Read the model definition and answer for the solid it produces. Units are mm, in the model's axes. Face numbers are marked on the shaded views. A direction names the side the tool comes from. Coordinates: 2 decimals unless noted, no trailing zeros. Loops run counter-clockwise (first coordinate to the right, second up) from the corner with the lowest first, then second, coordinate; pieces in that order, holes last. Notation, with made-up numbers: (36, 1.5) -> (90, 1.5) arc R12 ccw to (90, 7.5) -> close; hole circle Ø8 at (0.25, 2). An arc over 180 degrees is marked (long way). Answer as a JSON object with one key per item and string values. Group by question number.
1) Section C-C, the plane z = 54 is taken. Give the vertices of the cut face in (x, y).
2) Determine the mould class of the marked faces 4 and 5 for opening direction Y: released by +Y, released by -Y, zero draft, split by the parting line, or undercut.
3) Section A-A, the plane y = -15 is taken. Give the vertices of the cut face in (x, z).
4) Consider probe 1 along Z at (x, y) = (3, -10); probe 2 along Y at (x, z) = (1.5, 76); probe 3 along X at (y, z) = (-70, 68.5). Determine where each line is inside the solid, lowest interval first. Write a range as [from, to].
5) Flat-ended cylindrical pins translate along their axes: P1, Ø4, axis at y = -55, z = 77.5, coming from the +X side; P2, Ø12, axis at x = 6, y = -75.5, coming from the +Z side; P3, Ø24, axis at y = -50, z = 78.5, coming from the -X side; P4, Ø1, axis at x = 7, y = -22, coming from the +Z side. Find the tip coordinate at first contact, or state that the pin passes through.
6) Section D-D, the plane y = -54 is taken. Give the vertices of the cut face in (x, z).
7) Which of the six approach directions +Z, -Z, +X, -X, +Y, -Y give full straight-line access (tool end or side, diameter ignored) to the marked faces 1, 2 and 3?
8) Section B-B, the plane x = 7.25 is taken. Give the vertices of the cut face in (y, z).
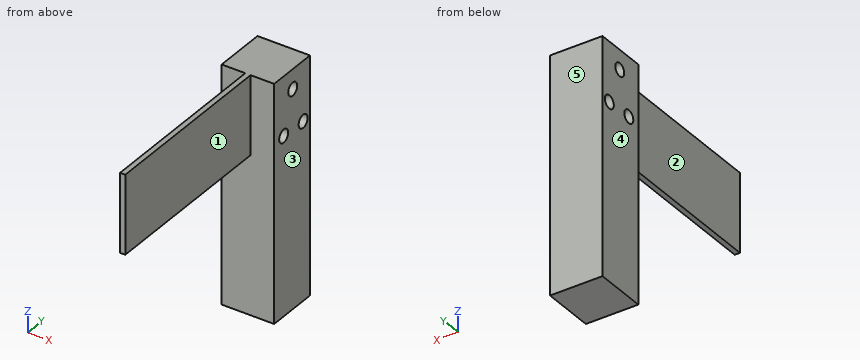
from build123d import *

# Parameters (mm, degrees)
F1_DEPTH = 20
F2_W     = 2
F2_H     = 30
F3_DEPTH = 90
F4_R     = 2.5
F5_DEPTH = 25


with BuildPart() as f1:
    # F0 (on Front) → F1 (new body)
    with BuildSketch(Plane.XZ):
        Polygon((0, 90), (0, 0), (20, 0), (20, 90), (11, 90), (11, 60), (9, 60), (9, 90), align=None)
    extrude(amount=F1_DEPTH)

    # F2 (on face) → F3 (join)
    with BuildSketch(Plane(origin=(0, 0, 0), x_dir=(-1, 0, 0), z_dir=(0, 1, 0))):
        with Locations((-10, 75)):
            Rectangle(F2_W, F2_H)
    extrude(amount=-F3_DEPTH)

    # F4 (on face) → F5 (cut)
    with BuildSketch(Plane(origin=(0, 0, 0), x_dir=(0, -1, 0), z_dir=(-1, 0, 0))):
        with Locations((9.6371909603, 82.499884069)):
            Circle(F4_R)
        with Locations((3.8047288544, 67.3352107406)):
            Circle(F4_R)
        with Locations((14.7008737549, 67.6194578409)):
            Circle(F4_R)
    extrude(amount=-F5_DEPTH, mode=Mode.SUBTRACT)


solid = f1.part
Determined:
{
 "1": {"outline": "(0, -20) -> (20, -20) -> (20, 0) -> (0, 0) -> close"},
 "2": {"face 4": "zero draft", "face 5": "released by +Y"},
 "3": {"outline": "(0, 0) -> (20, 0) -> (20, 65.14) -> (0, 65.14) -> close; (0, 70.1) -> (20, 70.1) -> (20, 90) -> (0, 90) -> close"},
 "4": {"probe 1": "[0, 80.03], [84.97, 90]", "probe 2": "[-20, 0]", "probe 3": "[9, 11]"},
 "5": {"P1": "x = 11", "P2": "z = 90", "P3": "x = 9", "P4": "through"},
 "6": {"outline": "(9, 60) -> (11, 60) -> (11, 90) -> (9, 90) -> close"},
 "7": {"face 1": "+Z, -Z, +X, -Y", "face 2": "+Z, -Z, -X, -Y", "face 3": "+Z, -Z, +X, +Y, -Y"},
 "8": {"outline": "(-20, 0) -> (0, 0) -> (0, 90) -> (-20, 90) -> close; hole circle Ø5 at (-14.7, 67.62); hole circle Ø5 at (-9.64, 82.5); hole circle Ø5 at (-3.8, 67.34)"}
}
